from build123d import *

# Parameters (mm, degrees)
SFAZOWANIE1_SIZE           = 1
SFAZOWANIE1_SIZE2          = 0.577350269
SFAZOWANIE1_PART_2_SIZE    = 1
SFAZOWANIE1_PART_2_SIZE2   = 0.577350269
WYTNIJ_WYCI_GNI_CIE1_START = -4.5
SZKIC2_R                   = 6
SZKIC2_R_2                 = 5.75
WYTNIJ_WYCI_GNI_CIE1_DEPTH = 1


with BuildPart() as part:
    # Szkic1 → Obrót1 (revolve)
    with BuildSketch(Plane.XY):
        Polygon((0, 0), (0, 8.5), (4, 8.5), (4, 6), (30, 6), (30, 0), align=None)
    revolve(axis=Axis((30, 0, 0), (-1, 0, 0)))

    # Sfazowanie1
    sfazowanie1_edges = [part.edges().sort_by_distance(p)[0] for p in [
        (30, -6, 0),
    ]]
    sfazowanie1_side = [part.faces().sort_by_distance(p)[0] for p in [
        (17, -6, 0),
    ]]
    chamfer(sfazowanie1_edges, length=SFAZOWANIE1_SIZE, length2=SFAZOWANIE1_SIZE2, reference=sfazowanie1_side[0])

    # Sfazowanie1 part 2
    sfazowanie1_part_2_edges = [part.edges().sort_by_distance(p)[0] for p in [
        (0, -8.5, 0),
    ]]
    sfazowanie1_part_2_side = [part.faces().sort_by_distance(p)[0] for p in [
        (0, 0, 0),
    ]]
    chamfer(sfazowanie1_part_2_edges, length=SFAZOWANIE1_PART_2_SIZE, length2=SFAZOWANIE1_PART_2_SIZE2, reference=sfazowanie1_part_2_side[0])

    # Szkic2 → Wytnij-wyciągnięcie1 (cut)
    with BuildSketch(Plane(origin=(30, 0, 0), x_dir=(0, 0, -1), z_dir=(1, 0, 0)).offset(WYTNIJ_WYCI_GNI_CIE1_START)):
        Circle(SZKIC2_R)
        Circle(SZKIC2_R_2, mode=Mode.SUBTRACT)
    extrude(amount=-WYTNIJ_WYCI_GNI_CIE1_DEPTH, mode=Mode.SUBTRACT)


solid = part.part
Model file for the job. Use its own axes, mm. A direction names the side the tool comes from. Give positions to 0.01 mm unless a question says otherwise; leave off trailing zeros. Loops run counter-clockwise (first coordinate to the right, second up) from the corner with the lowest first, then second, coordinate; pieces in that order, holes last.
1) Pull direction X, two halves, no side cores. Call faces 3 (the cylindrical face through (25.01, 5.7, 0.75)), 4 (the flat face through (30, 0, 0)), 5 (the cylindrical face through (27.27, 5.54, 2.3)): +X half, -X half, draft (parallel to the pull), parting line (faces both ways), or undercut.
2) Saw through at C-C (x = 7.75). Write the cut outline in (y, z).
3) Tool access for faces 1 (the cylindrical face through (2.313, 4.57, -7.167)), 2 (the cylindrical face through (14.39, 5.54, 2.3)): list every direction of +Z, -Z, +X, -X, +Y, -Y with a clear straight run to the whole face (end or side of a thin tool).
4) Saw through at D-D (x = 2). Write the cut outline in (y, z), plus the area to 3 significant figures.
5) Wall check: line 1 (X direction, y = -3.5, z = -5.5); line 2 (Z direction, x = 13.5, y = 1.25); line 3 (Z direction, x = 22.5, y = -5.25). Give the ranges that are in metal, low to high.
6) Saw through at A-A (z = 0). Write the cut outline in (x, y), plus the area to 3 significant figures.
7) Flat gauge pins, fed straight in: pin 1 Ø5 at (x, y) = (10.5, 4) entering from -Z; pin 2 Ø5 at (x, z) = (14, -3.5) entering from -Y; pin 3 Ø3 at (x, z) = (24, -5) entering from +Y. Where does each tip first touch, or does it go through?
Answer block:
1. face 3: undercut
1. face 4: +X half
1. face 5: draft
2. outline: circle Ø12 at (0, 0)
3. face 1: +X, -X
3. face 2: +X
4. outline: circle Ø17 at (0, 0)
4. area: 227 mm2
5. line 1: x = 0 to 4
5. line 2: z = -5.87 to 5.87
5. line 3: z = -2.9 to 2.9
6. outline: (0, -7.5) - (0.58, -8.5) - (4, -8.5) - (4, -6) - (24.5, -6) - (24.5, -5.75) - (25.5, -5.75) - (25.5, -6) - (29, -6) - (30, -5.42) - (30, 5.42) - (29, 6) - (25.5, 6) - (25.5, 5.75) - (24.5, 5.75) - (24.5, 6) - (4, 6) - (4, 8.5) - (0.58, 8.5) - (0, 7.5) - close
6. area: 378 mm2
7. pin 1: stops at z = -5.81
7. pin 2: stops at y = -5.92
7. pin 3: stops at y = 4.87
